from build123d import *

# Parameters (mm, degrees)
F0_W      = 26
F0_H      = 52
F1_DEPTH  = 84
F2_T      = -2
F4_DEPTH  = 3
F5_R      = 3.35
F6_DEPTH  = 3
F7_W      = 13
F7_H      = 13
F8_DEPTH  = 3
F9_W      = 16
F9_H      = 40
F10_DEPTH = 25


with BuildPart() as f1:
    # F0 (on Top) → F1 (new body)
    with BuildSketch(Plane.XY):
        Rectangle(F0_W, F0_H)
    extrude(amount=F1_DEPTH)

    # F2
    f2_openings = [f1.faces().sort_by_distance(p)[0] for p in [
        (0, 0, 0),
    ]]
    offset(amount=F2_T, openings=f2_openings)

    # F3 (on face) → F4 (cut)
    with BuildSketch(Plane(origin=(-13, 0, 0), x_dir=(0, -1, 0), z_dir=(-1, 0, 0))):
        with BuildLine():
            ThreePointArc((-21, 57), (0, 36), (21, 57))
            ThreePointArc((21, 57), (0, 78), (-21, 57))
        make_face()
        with BuildLine():
            Line((21, 0), (21, 57))
            ThreePointArc((21, 57), (0, 36), (-21, 57))
            Line((-21, 57), (-21, 0))
            Line((-21, 0), (21, 0))
        make_face()
    extrude(amount=-F4_DEPTH, mode=Mode.SUBTRACT)

    # F5 (on face) → F6 (cut)
    with BuildSketch(Plane.YZ.offset(13)):
        with Locations((0, 67)):
            Circle(F5_R)
        with Locations((0, 50)):
            Circle(F5_R)
    extrude(amount=-F6_DEPTH, mode=Mode.SUBTRACT)

    # F7 (on face) → F8 (cut)
    with BuildSketch(Plane(origin=(-13, 0, 0), x_dir=(0, -1, 0), z_dir=(-1, 0, 0))):
        with Locations((0, 67)):
            Rectangle(F7_W, F7_H)
        with Locations((0, 50)):
            Rectangle(F7_W, F7_H)
    extrude(amount=-F8_DEPTH, mode=Mode.SUBTRACT)

    # F9 (on face) → F10 (cut)
    with BuildSketch(Plane.XY.offset(84)):
        Rectangle(F9_W, F9_H)
    extrude(amount=-F10_DEPTH, mode=Mode.SUBTRACT)


solid = f1.part
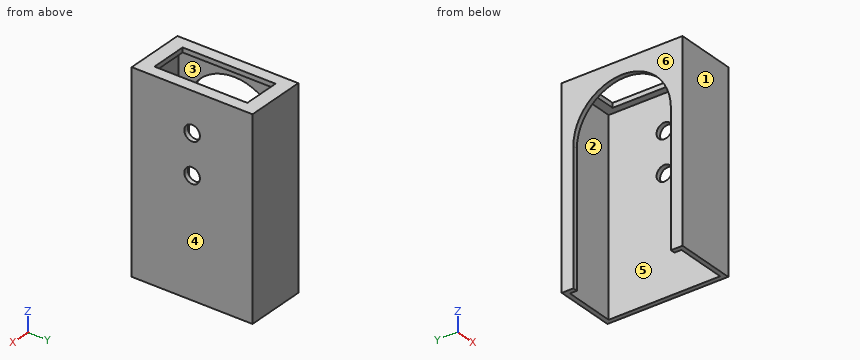
The listing builds one solid part. Answer for the finished solid, in the listing's coordinates (mm). Face numbers are marked on the shaded views. A direction names the side the tool comes from. Round coordinates to 2 decimals unless told otherwise and drop trailing zeros. Write each loop counter-clockwise with the first axis right and the second up, starting at its lowest first coordinate (ties: lowest second). Pieces come first, ordered by that corner, then holes. Notation, with made-up numbers: M 53,80 L 93,80 A29 ccw 93,105 Z; hole C 22.25,-18.75 d9. An arc over 180 degrees is marked long. Write each question's results on one line, items separated by ' | '. Start each with the question number.
Item 1: Find section A-A on x = -7. Write down the section's boundary in (y, z), and give its area (3 significant figures).
Item 2: Find section C-C on z = 50. Write down the section's boundary in (x, y).
Item 3: Find section D-D on y = 7.5. Write down the section's boundary in (x, z), and give its area (3 significant figures).
Item 4: Find section B-B on y = 0. Write down the section's boundary in (x, z), and give its area (3 significant figures).
Item 5: Which of the six approach directions +Z, -Z, +X, -X, +Y, -Y give full straight-line access (tool end or side, diameter ignored) to the marked faces 5 and 6?
Item 6: The mould has two halves that part along Y. Classify the marked faces 1, 2, 3 and 4: +Y half, -Y half, draft (parallel to the pull), parting line (faces both ways), or undercut.
Item 7: Straight lines are drawn through the part: probe 1 along Z at (x, y) = (12.2, 0); probe 2 along Y at (x, z) = (-0.75, 61); probe 3 along X at (y, z) = (-22, 58). For each, find the intervals that lie inside material, in ascending order.
Item 8: Given pin 1 Ø1 at (x, y) = (0, 19) entering from +Z; pin 2 Ø2 at (y, z) = (6.5, 36.5) entering from -X; pin 3 Ø6 at (x, y) = (5.5, 8.5) entering from -Z, each flat-ended and moving along its own axis, determine where each tip first touches the part or whether it passes through.
Answer block:
1) outline: M -26,0 L -24,0 L -24,82 L -20,82 L -20,84 L -26,84 Z; M 20,82 L 24,82 L 24,0 L 26,0 L 26,84 L 20,84 Z | area: 352 mm²
2) outline: M -13,-26 L 13,-26 L 13,-3.35 L 11,-3.35 L 11,-24 L -11,-24 L -11,-21 L -13,-21 Z; M -13,21 L -11,21 L -11,24 L 11,24 L 11,3.35 L 13,3.35 L 13,26 L -13,26 Z
3) outline: M -13,76.62 L -11,76.62 L -11,82 L -8,82 L -8,84 L -13,84 Z; M 8,82 L 11,82 L 11,0 L 13,0 L 13,84 L 8,84 Z | area: 195 mm²
4) outline: M -13,78 L -11,78 L -11,82 L -8,82 L -8,84 L -13,84 Z; M 8,82 L 11,82 L 11,70.35 L 13,70.35 L 13,84 L 8,84 Z; M 11,0 L 13,0 L 13,46.65 L 11,46.65 Z; M 11,53.35 L 13,53.35 L 13,63.65 L 11,63.65 Z | area: 165 mm²
5) face 5: -Z | face 6: +Z, -Z, -X, +Y, -Y
6) face 1: -Y half | face 2: undercut | face 3: undercut | face 4: draft
7) probe 1: z = 0 to 46.65, 53.35 to 63.65, 70.35 to 84 | probe 2: y = -26 to -24, 24 to 26 | probe 3: x = -13 to -11, 11 to 13
8) pin 1: passes through | pin 2: stops at x = 11 | pin 3: stops at z = 82
